```python
from build123d import *

# Parameters (mm, degrees)
F0_W     = 29
F0_H     = 27
F1_DEPTH = 2
F2_W     = 0.5
F2_H     = 27
F3_DEPTH = 10


with BuildPart() as f1:
    # F0 (on Top) → F1 (new body)
    with BuildSketch(Plane.XY):
        Rectangle(F0_W, F0_H)
    extrude(amount=F1_DEPTH)

    # F2 (on face) → F3 (join)
    with BuildSketch(Plane.XY.offset(2)):
        with Locations((-14.25, 0)):
            Rectangle(F2_W, F2_H)
        with Locations((-13.25, 0)):
            Rectangle(F2_W, F2_H)
        with Locations((-12.25, 0)):
            Rectangle(F2_W, F2_H)
        with Locations((-11.25, 0)):
            Rectangle(F2_W, F2_H)
        with Locations((-10.25, 0)):
            Rectangle(F2_W, F2_H)
        with Locations((-9.25, 0)):
            Rectangle(F2_W, F2_H)
        with Locations((-8.25, 0)):
            Rectangle(F2_W, F2_H)
        with Locations((-7.25, 0)):
            Rectangle(F2_W, F2_H)
        with Locations((-6.25, 0)):
            Rectangle(F2_W, F2_H)
        with Locations((-5.25, 0)):
            Rectangle(F2_W, F2_H)
        with Locations((-4.25, 0)):
            Rectangle(F2_W, F2_H)
        with Locations((-3.25, 0)):
            Rectangle(F2_W, F2_H)
        with Locations((-2.25, 0)):
            Rectangle(F2_W, F2_H)
        with Locations((-1.25, 0)):
            Rectangle(F2_W, F2_H)
        with Locations((-0.25, 0)):
            Rectangle(F2_W, F2_H)
        with Locations((0.75, 0)):
            Rectangle(F2_W, F2_H)
        with Locations((1.75, 0)):
            Rectangle(F2_W, F2_H)
        with Locations((2.75, 0)):
            Rectangle(F2_W, F2_H)
        with Locations((3.75, 0)):
            Rectangle(F2_W, F2_H)
        with Locations((4.75, 0)):
            Rectangle(F2_W, F2_H)
        with Locations((5.75, 0)):
            Rectangle(F2_W, F2_H)
        with Locations((6.75, 0)):
            Rectangle(F2_W, F2_H)
        with Locations((7.75, 0)):
            Rectangle(F2_W, F2_H)
        with Locations((8.75, 0)):
            Rectangle(F2_W, F2_H)
        with Locations((9.75, 0)):
            Rectangle(F2_W, F2_H)
        with Locations((10.75, 0)):
            Rectangle(F2_W, F2_H)
        with Locations((11.75, 0)):
            Rectangle(F2_W, F2_H)
        with Locations((12.75, 0)):
            Rectangle(F2_W, F2_H)
        with Locations((13.75, 0)):
            Rectangle(F2_W, F2_H)
    extrude(amount=F3_DEPTH)


solid = f1.part
```
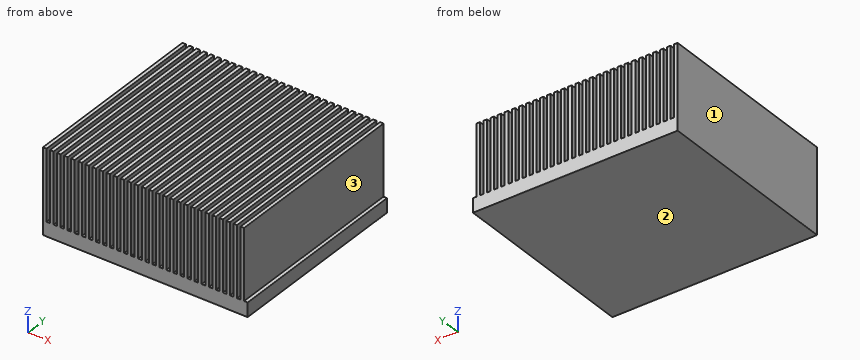
Read the model definition and answer for the solid it produces. Units are mm, in the model's axes. Face numbers are marked on the shaded views. Coordinates: 2 decimals unless noted, no trailing zeros. Answer as a JSON object with one key per item and string values. Group by question number.
Item 1: A flat-ended cylindrical pin translates along its axis: P1, Ø1, axis at y = 3, z = 8.5, coming from the +X side. Find the tip coordinate at first contact, or state that the pin passes through.
Item 2: Section A-A (z = 2.75) is taken. State how many separate pieces and enclosed holes the cut face has, plus the area to 4 significant figures.
Item 3: The mould has two halves that part along X. Classify the marked faces 1, 2 and 3: +X half, -X half, draft (parallel to the pull), parting line (faces both ways), or undercut.
Item 4: Consider probe 1 along Z at (x, y) = (-1.75, 3.5). Determine where the line is inside the solid, lowest interval first. Write a range as from..to.
Results are:
{
 "1": {"P1": "stops at x = 14"},
 "2": {"separate pieces": "29", "enclosed holes": "0", "area": "391.5 mm^2"},
 "3": {"face 1": "-X half", "face 2": "draft", "face 3": "+X half"},
 "4": {"probe 1": "z = 0..2"}
}
